Input: part model. Units: mm. Frame: model coordinates. A direction names the side the tool comes from. Round coordinates to 2 decimals unless told otherwise and drop trailing zeros. Order: outer loops, then holes, each group sorted by start corner. A loop starts at its lowest first (then second) coordinate and runs counter-clockwise, first axis right, second up. Notation, with made-up numbers: (40.5, 36) -> (62.5, 36) arc R25 ccw to (62.5, 72) -> close; hole circle Ø7 at (-32.75, 41). An arc over 180 degrees is marked (long way). Use a Markdown table: item, result.
from build123d import *

# Parameters (mm, degrees)
F0_W     = 914.4
F0_H     = 914.4
F1_DEPTH = 25.4
F2_R     = 13.97
F3_DEPTH = 57.15
F5_D     = 12.7


with BuildPart() as f1:
    # F0 (on Right) → F1 (new body)
    with BuildSketch(Plane.YZ):
        Rectangle(F0_W, F0_H)
    extrude(amount=F1_DEPTH)

    # F2 (on face) → F3 (join)
    with BuildSketch(Plane.YZ.offset(25.4)):
        Circle(F2_R)
    extrude(amount=F3_DEPTH)

    # F5 (through all)
    with Locations(Plane.YZ.offset(25.4)):
        with Locations((-128.5875, -273.05), (128.5875, -273.05), (128.5875, -336.55), (-128.5875, -336.55)):
            Hole(F5_D / 2)


solid = f1.part
1) Contact query for flat-ended pins moving along their axis: P1, Ø14.5, axis at y = -128.59, z = -273.05, coming from the +X side; P2, Ø1, axis at y = 125, z = 283, coming from the -X side. Output: stop coordinate, or through.
Answer key:
| item | result |
|---|---|
| P1 | stops at x = 25.4 |
| P2 | stops at x = 0 |
2) Cut plane C-C on y = -89.5. Return loops of the section in (x, z).
Answer key:
| item | result |
|---|---|
| outline | (0, -457.2) -> (25.4, -457.2) -> (25.4, 457.2) -> (0, 457.2) -> close |
3) Cut plane B-B on x = 38. Return loops of the section in (y, z), and give its area (3 significant figures).
Answer key:
| item | result |
|---|---|
| outline | circle Ø27.94 at (0, 0) |
| area | 613 mm^2 |
4) Ray query, probe 1 along Y at (x, z) = (6, -336); probe 2 along Y at (x, z) = (9, -273); probe 3 along X at (y, z) = (-54.5, 265). Return the intervals inside material, ascending.
Answer key:
| item | result |
|---|---|
| probe 1 | y = -457.2 to -134.91, -122.26 to 122.26, 134.91 to 457.2 |
| probe 2 | y = -457.2 to -134.94, -122.24 to 122.24, 134.94 to 457.2 |
| probe 3 | x = 0 to 25.4 |
5) Set-up query: faces 1 (the face through (53.57, -1.82, 13.85)), 2 (the face through (13, -6, -457.2)). Return all of +Z, -Z, +X, -X, +Y, -Y with unobstructed straight access to the full face (end or side cutting, diameter ignored); none if empty.
Answer key:
| item | result |
|---|---|
| face 1 | +X |
| face 2 | -Z, +X, -X, +Y, -Y |
6) Cut plane A-A on z = 0. Return loops of the section in (x, y).
Answer key:
| item | result |
|---|---|
| outline | (0, -457.2) -> (25.4, -457.2) -> (25.4, -13.97) -> (82.55, -13.97) -> (82.55, 13.97) -> (25.4, 13.97) -> (25.4, 457.2) -> (0, 457.2) -> close |
